Autodesk Inventor part; units mm, degrees
ref_plane "YZ Plane" through (0, 0, 0) normal (1, 0, 0) x (0, 1, 0)
ref_plane "XZ Plane" through (0, 0, 0) normal (0, 1, 0) x (-1, 0, 0)
ref_plane "XY Plane" through (0, 0, 0) normal (0, 0, 1) x (1, 0, 0)
sketch "Sketch1" plane through (0, 0, 0) normal (1, 0, 0) x (0, 1, 0)
  line L0 (11.5153, 6.5399) -> (13.2626, 6.1589)
  line L1 (-9.5192, 15.3385) -> (-9.5235, 15.3385)
  line L2 (-9.5235, 15.3385) -> (-9.5593, 15.3004)
  line L3 (-9.5593, 15.3004) -> (-9.5621, 15.2978)
  line L4 (-9.5621, 15.2978) -> (-9.9203, 14.9422)
  line L5 (-9.9203, 14.9422) -> (-10.6894, 13.5732)
  line L6 (-10.6894, 13.5732) -> (-10.9995, 11.6224)
  line L7 (-10.9995, 11.6224) -> (-10.4963, 9.7251)
  line L8 (-10.4963, 9.7251) -> (-9.5812, 8.4551)
  line L9 (-9.5812, 8.4551) -> (-9.1857, 8.1477)
  line L10 (-9.1857, 8.1477) -> (-8.6264, 7.7134)
  line L11 (-8.6264, 7.7134) -> (-5.7531, 5.4731)
  line L12 (-5.7531, 5.4731) -> (-3.125, 3.403)
  line L13 (-3.125, 3.403) -> (-2.6869, 3.0525)
  line L14 (-2.6869, 3.0525) -> (-2.235, 2.6918)
  line L15 (-2.235, 2.6918) -> (-0.8776, 1.6047)
  line L16 (-0.8776, 1.6047) -> (0.7277, 0.3271)
  line L17 (0.7277, 0.3271) -> (1.9751, -0.6483)
  line L18 (1.9751, -0.6483) -> (2.5659, -1.1004)
  line L19 (2.5659, -1.1004) -> (2.7096, -1.1969)
  line L20 (2.7096, -1.1969) -> (2.9464, -1.3595)
  line L21 (2.9464, -1.3595) -> (3.1338, -1.4865)
  line L22 (3.1338, -1.4865) -> (3.7002, -1.87)
  line L23 (3.7002, -1.87) -> (4.6441, -2.4873)
  line L24 (4.6441, -2.4873) -> (5.7068, -3.1426)
  line L25 (5.7068, -3.1426) -> (6.8158, -3.7623)
  line L26 (6.8158, -3.7623) -> (7.8978, -4.2754)
  line L27 (7.8978, -4.2754) -> (8.8818, -4.6132)
  line L28 (8.8818, -4.6132) -> (9.6959, -4.7021)
  line L29 (9.6959, -4.7021) -> (10.1645, -4.5726)
  line L30 (10.1645, -4.5726) -> (10.2664, -4.4735)
  line L31 (10.2664, -4.4735) -> (10.2776, -4.4608)
  line L32 (10.2776, -4.4608) -> (10.4693, -4.2627)
  line L33 (10.4693, -4.2627) -> (10.4289, -3.0664)
  line L34 (10.4289, -3.0664) -> (9.5831, -0.9963)
  line L35 (9.5831, -0.9963) -> (8.3108, 1.1754)
  line L36 (8.3108, 1.1754) -> (7.4706, 2.453)
  line L37 (7.4706, 2.453) -> (7.1838, 2.8747)
  line L38 (7.1838, 2.8747) -> (7.0213, 3.1134)
  line L39 (7.0213, 3.1134) -> (6.9248, 3.2557)
  line L40 (6.9248, 3.2557) -> (6.4739, 3.845)
  line L41 (6.4739, 3.845) -> (5.5001, 5.087)
  line L42 (5.5001, 5.087) -> (4.2278, 6.6872)
  line L43 (4.2278, 6.6872) -> (3.145, 8.041)
  line L44 (3.145, 8.041) -> (2.7851, 8.4906)
  line L45 (2.7851, 8.4906) -> (2.4351, 8.93)
  line L46 (2.4351, 8.93) -> (0.3586, 11.5615)
  line L47 (0.3586, 11.5615) -> (-1.8878, 14.4444)
  line L48 (-1.8878, 14.4444) -> (-2.3231, 15.0083)
  line L49 (-2.3231, 15.0083) -> (-2.6305, 15.402)
  line L50 (-2.6305, 15.402) -> (-3.9025, 16.3189)
  line L51 (-3.9025, 16.3189) -> (-5.8001, 16.8218)
  line L52 (-5.8001, 16.8218) -> (-7.7486, 16.5119)
  line L53 (-7.7486, 16.5119) -> (-9.1212, 15.7449)
  line L54 (-9.1212, 15.7449) -> (-9.475, 15.3842)
  line L55 (-9.475, 15.3842) -> (-9.4793, 15.3816)
  line L56 (-9.4793, 15.3816) -> (-9.5167, 15.3435)
  line L57 (-9.5167, 15.3435) -> (-9.5192, 15.3385)
extrude "Extrusion27" add sketch "Sketch1" along normal blind 0.25
sketch "Sketch7" plane through (0, 0, 0) normal (-1, 0, 0) x (0, 0, 1)
  circle A0 centre (11.7567, -6.0872) radius 5
  circle A1 centre (11.7567, -6.0872) radius 0.5
  point P0 (0, 0)
  dimension "d91" = 10
  dimension "d92" = 1
extrude "Extrusion30" [suppressed]
properties part number "Sticker7"
Could you check a few things on this model? Use its own coordinates, in mm. Coordinates: 2 decimals unless noted, no trailing zeros. Write each loop counter-clockwise with the first axis right and the second up, starting at its lowest first coordinate (ties: lowest second). Pieces come first, ordered by that corner, then holes. Notation, with made-up numbers: M -36,47 L -16,47 A18 cw -16,69 Z; hole C -3,76 d4. An arc over 180 degrees is marked long. One line per question, with ' | ' between items.
1) Imagine slicing it at A-A, the plane z = 2. Write out the boundary of the cut face in (x, y), and give its area (3 significant figures).
Checks:
outline: M 0,-1.37 L 0.25,-1.37 L 0.25,7.77 L 0,7.77 Z | area: 2.28 mm²
2) I need wall thicknesses on probe 1 along Y at (x, z) = (0.1, -1); probe 2 along Z at (x, y) = (0.2, 8.75); probe 3 along Y at (x, z) = (0.1, -0.75). Which ranges of each line are inside material? Lowest first, please. Write a range as [from, to].
Checks:
probe 1: [2.43, 9.58] | probe 2: [-4.57, 0.43] | probe 3: [2.11, 9.44]
3) Imagine slicing it at B-B, the plane y = -6.75. Write out the boundary of the cut face in (x, z), and give its area (3 significant figures).
Checks:
outline: M 0,6.25 L 0.25,6.25 L 0.25,16.67 L 0,16.67 Z | area: 2.61 mm²
